Study the drawing (mm; zero at the part's minimum x, y, z) and answer. A direction names the side the tool comes from. Give positions to 0.01 mm unless a question says otherwise; leave off trailing zeros. Order: outer loops, then holes, each group sorted by start corner. A loop starts at its lowest first (then second) coordinate and runs counter-clockwise, first axis right, second up. Notation, with made-up numbers: (31, -31.5) - (87, -31.5) arc R22 ccw to (87, -2.5) - close; hole circle Ø6 at (-30.75, -2.75). An arc over 180 degrees is marked (long way). Return JSON: item names as keys, results as strings.
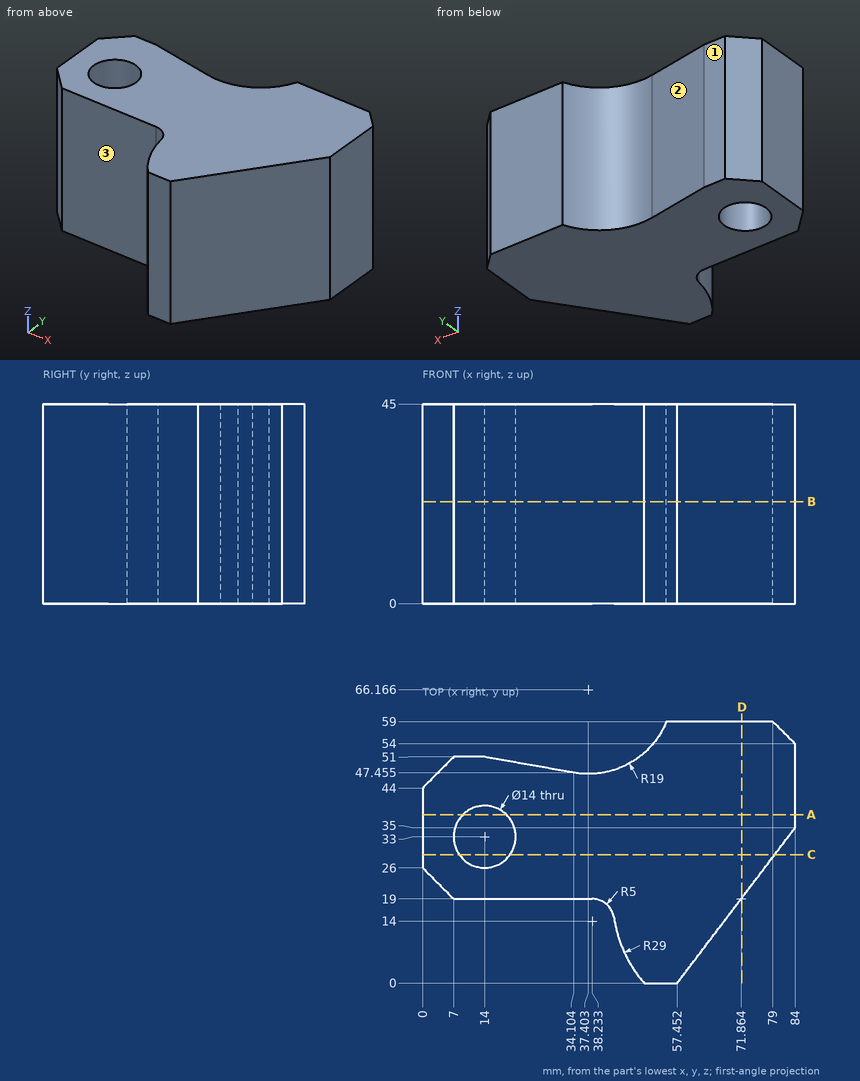
Q1. A cutting plane is placed at D-D (x = 72). Write down the section's boundary in (y, z), and give its area (3 significant figures).
Values:
{"outline": "(19.18, 0) - (59, 0) - (59, 45) - (19.18, 45) - close", "area": "1,790 mm²"}
Q2. Consider L1, parallel to X at y = 15, z = 43.5; L2, parallel to Y at x = 19.5, z = 34; L3, parallel to Y at x = 32, z = 13 (1 decimal). Determine where each line is inside the solid, lowest interval first.
Values:
{"L1": "x = 43.13 to 68.83", "L2": "y = 19 to 28.67, 37.33 to 50.03", "L3": "y = 19 to 47.8"}
Q3. For the marked faces 1, 2 and 3, determine the directions among +Z, -Z, +X, -X, +Y, -Y from which every point of the face is accessible in a straight line to the end or side of a thin tool.
Values:
{"face 1": "+Z, -Z, -X, +Y", "face 2": "+Z, -Z, +Y", "face 3": "+Z, -Z, -X, -Y"}
Q4. Given pin 1 (3 mm diameter, centred on x = 25.5, z = 8.5, fed in from +Y); pin 2 (1 mm diameter, centred on y = 11.5, z = 30.5, fed in from +X) (1 decimal); pin 3 (25 mm diameter, centred on x = 29.5, z = 12.5, fed in from -Y); pin 4 (18 mm diameter, centred on x = 14, y = 33, fed in from -Z), each flat-ended and moving along its own axis, determine where each tip first touches the part or whether it passes through.
Values:
{"pin 1": "stops at y = 49.24", "pin 2": "stops at x = 66.6", "pin 3": "stops at y = 17.29", "pin 4": "stops at z = 0"}
Q5. A cutting plane is placed at C-C (y = 29). Write down the section's boundary in (x, z) (1 decimal).
Values:
{"outline": "(0, 0) - (8.3, 0) - (8.3, 45) - (0, 45) - close; (19.7, 0) - (79.4, 0) - (79.4, 45) - (19.7, 45) - close"}
Q6. A cutting plane is placed at B-B (z = 23). Write down the section's boundary in (x, y) (1 decimal), and give its area (3 significant figures).
Values:
{"outline": "(0, 26) - (7, 19) - (38.2, 19) arc R5 cw to (43.2, 14.7) arc R29 ccw to (50, 0) - (57.5, 0) - (84, 35) - (84, 54) - (79, 59) - (55, 59) arc R19 cw to (34.1, 47.5) - (14, 51) - (7, 51) - (0, 44) - close; hole circle Ø14 at (14, 33)", "area": "2,930 mm²"}
Q7. A cutting plane is placed at A-A (y = 38). Write down the section's boundary in (x, z), and give its area (3 significant figures).
Values:
{"outline": "(0, 0) - (9.1, 0) - (9.1, 45) - (0, 45) - close; (18.9, 0) - (84, 0) - (84, 45) - (18.9, 45) - close", "area": "3,340 mm²"}
